Check sheet for the drawn part. Datum: minimum x, y, z corner. Units: mm. A direction names the side the tool comes from. Give positions to 0.01 mm unless a question says otherwise; leave off trailing zeros. Order: outer loops, then holes, each group sorted by start corner. A loop starts at its lowest first (then second) coordinate and runs counter-clockwise, first axis right, second up.
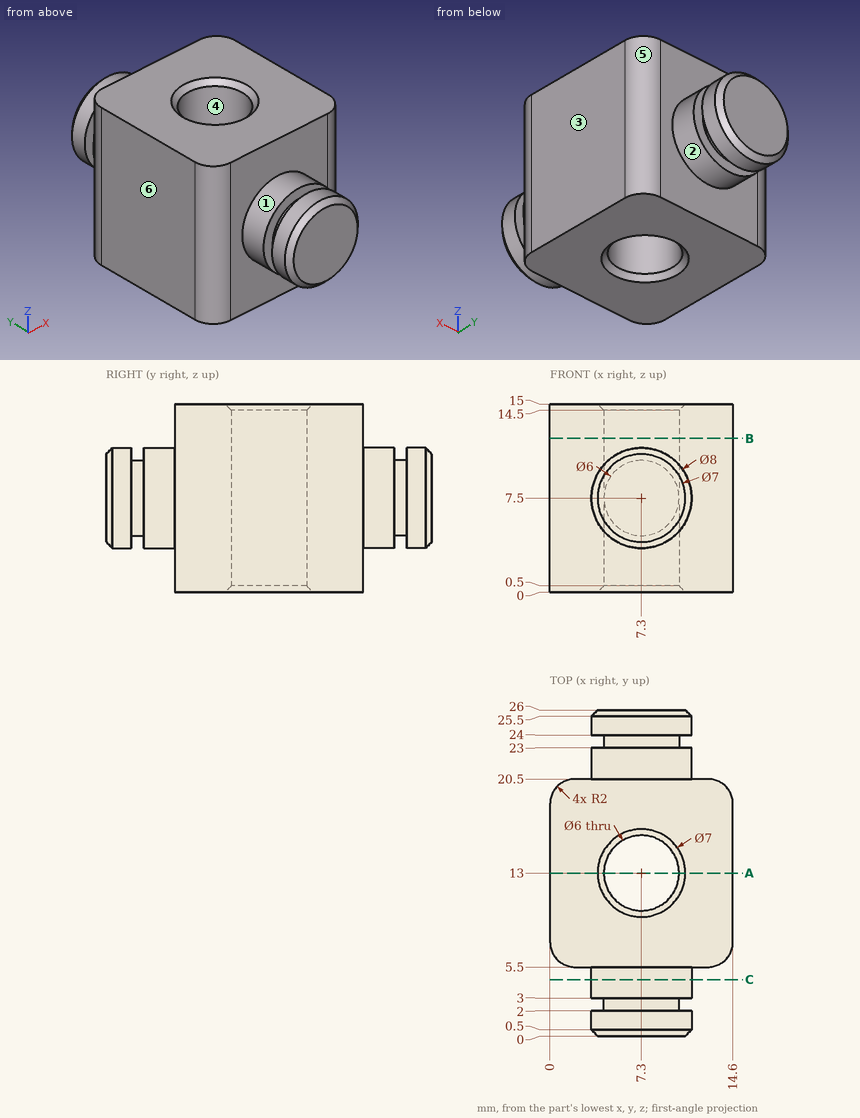
Item 1: Sectioned sample at C-C (y = 4.5). Enter the section's corners in (x, z), and give its area (3 significant figures).
Reported:
outline: circle Ø8 at (7.3, 7.5)
area: 50.3 mm2
Item 2: Gauge pin test, flat ends, axial feed: pin 1 (5 mm diameter, centred on y = 11.5, z = 3, fed in from -X); pin 2 (1 mm diameter, centred on y = 4, z = 4.5, fed in from -X); pin 3 (3 mm diameter, centred on y = 4.5, z = 9.5, fed in from +X). Record the tip position at first contact, or that the pin passes through.
Reported:
pin 1: stops at x = 0
pin 2: stops at x = 4.18
pin 3: stops at x = 13.92
Item 3: Draft check along X on the marked faces 4, 5 and 6. Enter one of: released by +X, released by -X, zero draft, split by the parting line, or undercut.
Reported:
face 4: undercut
face 5: released by +X
face 6: released by -X
Item 4: Sectioned sample at A-A (y = 13). Enter the section's corners in (x, z).
Reported:
outline: (0, 0) - (3.8, 0) - (4.3, 0.5) - (4.3, 14.5) - (3.8, 15) - (0, 15) - close; (10.3, 0.5) - (10.8, 0) - (14.6, 0) - (14.6, 15) - (10.8, 15) - (10.3, 14.5) - close
Item 5: Sectioned sample at B-B (z = 12.25). Enter the section's corners in (x, y), and give its area (3 significant figures).
Reported:
outline: (0, 7.5) arc R2 ccw to (2, 5.5) - (12.6, 5.5) arc R2 ccw to (14.6, 7.5) - (14.6, 18.5) arc R2 ccw to (12.6, 20.5) - (2, 20.5) arc R2 ccw to (0, 18.5) - close; hole circle Ø6 at (7.3, 13)
area: 187 mm2
Item 6: Scan lines: L1, parallel to Y at x = 7.3, z = 5.5; L2, parallel to Y at x = 7.5, z = 2.75; L3, parallel to Y at x = 2.5, z = 10.25. Record each from-to range of solid material in increasing order.
Reported:
L1: y = 0 to 10, 16 to 26
L2: y = 5.5 to 10.01, 15.99 to 20.5
L3: y = 5.5 to 20.5
Item 7: Set-up check for the marked faces 1, 2 and 3: record each of +Z, -Z, +X, -X, +Y, -Y from which the full face is reachable in a straight line by a thin tool's end or side.
Reported:
face 1: -Y
face 2: +Y
face 3: +Z, -Z, +X, +Y, -Y
